```python
from build123d import *

# Parameters (mm, degrees)
SKETCH1_R            = 110
SKETCH1_R_2          = 90
BOSS_EXTRUDE1_DEPTH  = 3.175
M3_CLEARANCE_HOLE1_D = 3.4


with BuildPart() as part:
    # Sketch1 → Boss-Extrude1 (new body)
    with BuildSketch(Plane(origin=(0, 0, 0), x_dir=(1, 0, 0), z_dir=(0, 1, 0))):
        with Locations(Location((0, 0, 0), (0, 0, 270))):
            Circle(SKETCH1_R)
        with Locations(Location((0, 0, 0), (0, 0, 270))):
            Circle(SKETCH1_R_2, mode=Mode.SUBTRACT)
    extrude(amount=BOSS_EXTRUDE1_DEPTH)

    # M3 Clearance Hole1 (through all)
    with Locations(Plane(origin=(0, 3.175, 0), x_dir=(1, 0, 0), z_dir=(0, 1, 0))):
        with Locations((0, 105), (52.5, 90.932667397), (90.932667397, 52.5), (105, 0), (90.932667397, -52.5), (52.5, -90.932667397), (0, -105), (-52.5, -90.932667397), (-90.932667397, -52.5), (-105, 0), (-90.932667397, 52.5), (-52.5, 90.932667397)):
            Hole(M3_CLEARANCE_HOLE1_D / 2)


solid = part.part
```
Source: CAD feature listing. Evaluate the final solid. Frame: model axes, mm. Round coordinates to 2 decimals unless told otherwise and drop trailing zeros. Loops run counter-clockwise (first coordinate to the right, second up) from the corner with the lowest first, then second, coordinate; pieces in that order, holes last.
1. Ray query, L1, parallel to Z at x = -53.5, y = 0.8; L2, parallel to X at y = 1.5, z = -52.5. Return the intervals inside material, ascending.
2. Section query B-B on z = -86. Output: boundary loops of the cut face in (x, y) (3 decimals), and give its area (3 significant figures).
3. Section query C-C on y = 0.8. Give the number of separate pieces and of enclosed holes in the cut face, and give its area (3 significant figures).
4. Section query A-A on x = 13. Output: boundary loops of the cut face in (y, z) (3 decimals).
5. Mould query, pull axis Z, two halves, no side actions, for faces 1 (the flat face through (-89, 3.175, -17)), 2 (the cylindrical face through (-34.471, 1.565, 83.137)), 3 (the cylindrical face through (-97.59, 1.57, 50.76)). Classes: released by +Z, released by -Z, zero draft, split by the parting line, or undercut.
Answers below:
1. L1: z = -96.11 to -92.31, -89.56 to -72.37, 72.37 to 89.56, 92.31 to 96.11
1. L2: x = -96.66 to -92.63, -89.23 to -73.1, 73.1 to 89.23, 92.63 to 96.66
2. outline: (-68.586, 0) - (-26.533, 0) - (-26.533, 3.175) - (-68.586, 3.175) - close; (26.533, 0) - (68.586, 0) - (68.586, 3.175) - (26.533, 3.175) - close
2. area: 267 mm2
3. separate pieces: 1
3. enclosed holes: 13
3. area: 12,500 mm2
4. outline: (0, -109.229) - (3.175, -109.229) - (3.175, -89.056) - (0, -89.056) - close; (0, 89.056) - (3.175, 89.056) - (3.175, 109.229) - (0, 109.229) - close
5. face 1: zero draft
5. face 2: undercut
5. face 3: split by the parting line
